Design review of the part shown in the three views and the two pictorial views. Dimensions are in mm from the part's minimum x, y and z. A direction names the side the tool comes from. Round coordinates to 2 decimals unless told otherwise and drop trailing zeros. Loops run counter-clockwise (first coordinate to the right, second up) from the corner with the lowest first, then second, coordinate; pieces in that order, holes last.
1) Tool access review of the marked faces 1, 2 and 3: name each direction out of +Z, -Z, +X, -X, +Y, -Y from which nothing blocks a thin tool from reaching the whole face with its end or side.
2) Take a section at D-D (z = 3.75). State the section outline as (x, y) points.
3) Insertion check: pin 1 (3.5 mm diameter, centred on x = 10, z = 3.75, fed in from +Y); pin 2 (11 mm diameter, centred on x = 8, z = 8.5, fed in from -Y); pin 3 (16.5 mm diameter, centred on x = 18, z = 28, fed in from +Y); pin 4 (6 mm diameter, centred on x = 39, y = 25, fed in from +Z). Each pin has a flat end and moves straight along its axis. Give the tip position at first contact, or say it passes through.
4) Take a section at A-A (z = 24.5). State the section outline as (x, y) points.
5) Take a section at B-B (x = 40). State the section outline as (y, z) points, then the cut area to 3 significant figures.
6) Take a section at C-C (y = 23). State the section outline as (x, z) points.
7) Wall thickness on L1, parallel to X at y = 30.4, z = 3.75; L2, parallel to X at y = 0.7, z = 24.5; L3, parallel to Z at x = 40, y = 0.6: over which ranges is each line inside the solid? List them lowest first.
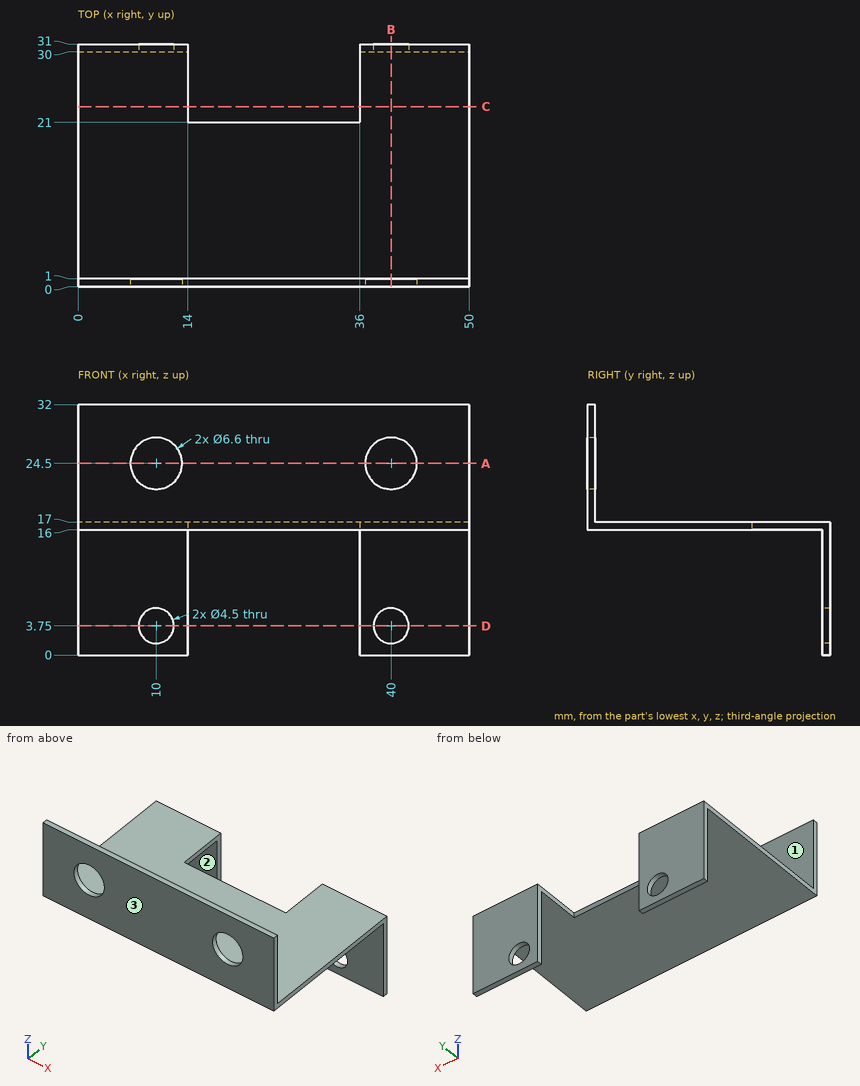
Response:
1. face 1: +Z, +X, -X, +Y
1. face 2: -Z, +X, -X, -Y
1. face 3: +Z, -Z, +X, -X, -Y
2. outline: (0, 30) - (7.75, 30) - (7.75, 31) - (0, 31) - close; (12.25, 30) - (14, 30) - (14, 31) - (12.25, 31) - close; (36, 30) - (37.75, 30) - (37.75, 31) - (36, 31) - close; (42.25, 30) - (50, 30) - (50, 31) - (42.25, 31) - close
3. pin 1: passes through
3. pin 2: stops at y = 30
3. pin 3: stops at y = 1
3. pin 4: stops at z = 17
4. outline: (0, 0) - (6.7, 0) - (6.7, 1) - (0, 1) - close; (13.3, 0) - (36.7, 0) - (36.7, 1) - (13.3, 1) - close; (43.3, 0) - (50, 0) - (50, 1) - (43.3, 1) - close
5. outline: (0, 16) - (30, 16) - (30, 6) - (31, 6) - (31, 17) - (1, 17) - (1, 21.2) - (0, 21.2) - close; (0, 27.8) - (1, 27.8) - (1, 32) - (0, 32) - close; (30, 0) - (31, 0) - (31, 1.5) - (30, 1.5) - close
5. area: 50.9 mm2
6. outline: (0, 16) - (14, 16) - (14, 17) - (0, 17) - close; (36, 16) - (50, 16) - (50, 17) - (36, 17) - close
7. L1: x = 0 to 7.75, 12.25 to 14, 36 to 37.75, 42.25 to 50
7. L2: x = 0 to 6.7, 13.3 to 36.7, 43.3 to 50
7. L3: z = 16 to 21.2, 27.8 to 32
